from build123d import *

# Parameters (mm, degrees)
ESBO_O1_W                = 22.8
ESBO_O1_H                = 12.3
RESSALTO_EXTRUS_O1_DEPTH = 16
ESBO_O2_W                = 32.4
ESBO_O2_H                = 12.3
RESSALTO_EXTRUS_O2_DEPTH = 2.35
ESBO_O3_W                = 22.8
ESBO_O3_H                = 12.3
RESSALTO_EXTRUS_O3_DEPTH = 4.25
CORTE_EXTRUS_O1_DEPTH    = 4.25
RESSALTO_EXTRUS_O4_DEPTH = 4.35
ESBO_O6_R                = 2.3
RESSALTO_EXTRUS_O5_DEPTH = 2.7


with BuildPart() as part:
    # Esboço1 → Ressalto-extrusão1 (new body)
    with BuildSketch(Plane(origin=(0, 0, 0), x_dir=(1, 0, 0), z_dir=(0, 1, 0))):
        Rectangle(ESBO_O1_W, ESBO_O1_H)
    extrude(amount=RESSALTO_EXTRUS_O1_DEPTH)

    # Esboço2 → Ressalto-extrusão2 (add)
    with BuildSketch(Plane(origin=(0, 16, 0), x_dir=(1, 0, 0), z_dir=(0, 1, 0))):
        Rectangle(ESBO_O2_W, ESBO_O2_H)
    extrude(amount=RESSALTO_EXTRUS_O2_DEPTH)

    # Esboço3 → Ressalto-extrusão3 (add)
    with BuildSketch(Plane(origin=(0, 18.35, 0), x_dir=(-1, 0, 0), z_dir=(0, 1, 0))):
        Rectangle(ESBO_O3_W, ESBO_O3_H)
    extrude(amount=RESSALTO_EXTRUS_O3_DEPTH)

    # Esboço4 → Corte-extrusão1 (cut)
    with BuildSketch(Plane(origin=(0, 18.35, 0), x_dir=(1, 0, 0), z_dir=(0, 1, 0))):
        with BuildLine():
            Line((16.2, 0), (16.2, 0.58))
            Line((16.2, 0.58), (14.675271386, 0.58))
            ThreePointArc((14.675271386, 0.58), (12.75, 0), (14.675271386, -0.58))
            Line((14.675271386, -0.58), (16.2, -0.58))
            Line((16.2, -0.58), (16.2, 0))
        make_face()
        with BuildLine():
            Line((-16.2, 0.58), (-14.675271386, 0.58))
            ThreePointArc((-14.675271386, 0.58), (-12.75, 0), (-14.675271386, -0.58))
            Line((-14.675271386, -0.58), (-16.2, -0.58))
            Line((-16.2, -0.58), (-16.2, 0))
            Line((-16.2, 0), (-16.2, 0.58))
        make_face()
    extrude(amount=-CORTE_EXTRUS_O1_DEPTH, mode=Mode.SUBTRACT)

    # Esboço5 → Ressalto-extrusão4 (add)
    with BuildSketch(Plane(origin=(0, 22.6, 0), x_dir=(1, 0, 0), z_dir=(0, 1, 0))):
        with BuildLine():
            ThreePointArc((0.315959416, 2.381386118), (-11.4, 0), (0.315959416, -2.381386118))
            ThreePointArc((0.315959416, -2.381386118), (3.351959063, 0), (0.315959416, 2.381386118))
        make_face()
    extrude(amount=RESSALTO_EXTRUS_O4_DEPTH)

    # Esboço6 → Ressalto-extrusão5 (add)
    with BuildSketch(Plane(origin=(0, 26.95, 0), x_dir=(1, 0, 0), z_dir=(0, 1, 0))):
        with Locations(Location((-5.3, 0, 0), (0, 0, 90))):
            Circle(ESBO_O6_R)
    extrude(amount=RESSALTO_EXTRUS_O5_DEPTH)


solid = part.part
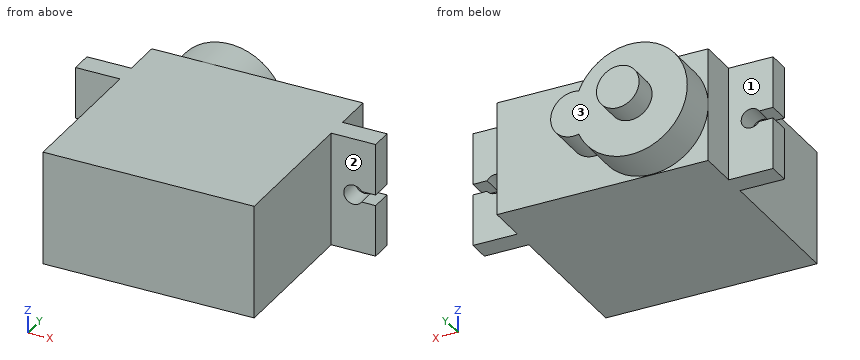
For this review, take the finished solid that the model builds, in its own axes (mm). Face numbers are marked on the shaded views. A direction names the side the tool comes from. Give positions to 0.01 mm unless a question says otherwise; leave off trailing zeros. Write each loop counter-clockwise with the first axis right and the second up, starting at its lowest first coordinate (ties: lowest second). Pieces come first, ordered by that corner, then holes. Notation, with made-up numbers: (10.25, 32.5) -> (31.25, 32.5) arc R24 cw to (31.25, 43.5) -> close; hole circle Ø2 at (88, 25.25). An arc over 180 degrees is marked (long way). Use CSV: the item, a comma, the result in double quotes.
Q1. Take a section at A-A, the plane x = -13.8. Write out the cut boundary in (y, z), then the cut area to 3 significant figures.
Conclusion:
outline,"(16, -6.15) -> (18.35, -6.15) -> (18.35, -1.05) -> (16, -1.05) -> close; (16, 1.05) -> (18.35, 1.05) -> (18.35, 6.15) -> (16, 6.15) -> close"
area,"24.0 mm2"
Q2. For P1, Ø1.3, axis at y = 20, z = 1, coming from the -X side; P2, Ø2, axis at y = 21, z = -2.5, coming from the +X side; P3, Ø2.5, axis at x = -13.8, z = 0, coming from the +Y side, all flat-tipped, find the tip position at first contact; note any pin that passes through.
Conclusion:
P1,"x = -11.4"
P2,"x = 11.4"
P3,"y = 18.35"
Q3. Tool access review of the marked faces 1, 2 and 3: name each direction out of +Z, -Z, +X, -X, +Y, -Y from which nothing blocks a thin tool from reaching the whole face with its end or side.
Conclusion:
face 1,"+Z, -Z, -X, +Y"
face 2,"+Z, -Z, +X, -Y"
face 3,"+Y"
Q4. To check wall thickness, follow probe 1 along Z at (x, y) = (-13.8, 17.3); probe 2 along X at (y, z) = (10.5, -2.75); probe 3 along Y at (x, z) = (11, -2). State the ranges of each line that lie inside material, in increasing order. Write a range as [from, to].
Conclusion:
probe 1,"[-6.15, -1.05], [1.05, 6.15]"
probe 2,"[-11.4, 11.4]"
probe 3,"[0, 22.6]"
Q5. Take a section at B-B, the plane x = -5.3. Write out the cut boundary in (y, z).
Conclusion:
outline,"(0, -6.15) -> (22.6, -6.15) -> (22.6, -6.1) -> (26.95, -6.1) -> (26.95, -2.3) -> (29.65, -2.3) -> (29.65, 2.3) -> (26.95, 2.3) -> (26.95, 6.1) -> (22.6, 6.1) -> (22.6, 6.15) -> (0, 6.15) -> close"
Q6. Take a section at C-C, the plane z = 3. Write out the cut boundary in (x, y).
Conclusion:
outline,"(-16.2, 16) -> (-11.4, 16) -> (-11.4, 0) -> (11.4, 0) -> (11.4, 16) -> (16.2, 16) -> (16.2, 18.35) -> (11.4, 18.35) -> (11.4, 22.6) -> (0.01, 22.6) -> (0.01, 26.95) -> (-10.61, 26.95) -> (-10.61, 22.6) -> (-11.4, 22.6) -> (-11.4, 18.35) -> (-16.2, 18.35) -> close"
Q7. Take a section at D-D, the plane y = 22. Write out the cut boundary in (x, z).
Conclusion:
outline,"(-11.4, -6.15) -> (11.4, -6.15) -> (11.4, 6.15) -> (-11.4, 6.15) -> close"
